For this review, take the finished solid that the model builds, in its own axes (mm). A direction names the side the tool comes from. Give positions to 0.01 mm unless a question says otherwise; leave off trailing zeros. Loops run counter-clockwise (first coordinate to the right, second up) from the corner with the lowest first, then second, coordinate; pieces in that order, holes last. Notation, with made-up numbers: (-27, -35.75) -> (2, -35.75) arc R21 ccw to (2, -2.75) -> close; hole circle Ø4 at (36.25, 52). An arc over 180 degrees is marked (long way). Answer as CSV lines item,"result". Start each with the question number.
Item 1: Machinability: for faces 1 (the face through (0, -1.5, 12)), 2 (the face through (12.93, 3.9, 11.93)), 3 (the face through (-0.147, 2.197, 2.317)), which of the approach directions +Z, -Z, +X, -X, +Y, -Y give a long, thin tool a straight path to every point of the face, cutting with its end or side? Answer none if there is none.
Item 2: For L1, parallel to Y at x = 3, z = 18; L2, parallel to Z at x = -15.5, y = -8.75; L3, parallel to Z at x = 1, y = 2, list the stretches that pass through material, from the lowest coordinate up. Write a range as from..to.
Item 3: Add section B-B on z = 15. State the section outline as (x, y) points.
Item 4: Clearance check with flat-ended pins moving along their axes: P1, Ø4, axis at x = 10, z = 15.5, coming from the +Y side; P2, Ø5, axis at y = 3, z = 6.5, coming from the +X side; P3, Ø4, axis at y = -1, z = 11.5, coming from the -X side. State where each tip first meets the part, or that it passes through.
Item 5: Add section D-D on y = 5.25. State the section outline as (x, z) points.
Item 6: The part is to be moulded in two halves that separate along Y. For faces 4 (the face through (0, 5, 0.2)), 5 (the face through (-12.93, -3.9, 11.93)), 6 (the face through (-0.147, -2.217, 22.731)), say which applies: +Y half, -Y half, draft (parallel to the pull), parting line (faces both ways), or undercut.
Item 7: Add section C-C on x = -11. State the section outline as (y, z) points, plus the area to 3 significant figures.
```python
from build123d import *

# Parameters (mm, degrees)
F0_W     = 21
F0_H     = 3
F1_DEPTH = 25
F2_SIZE  = 2
F3_SIZE  = 2
F4_R     = 0.99999
F0_W_2   = 36.543905735
F0_H_2   = 20.3890502453
F5_DEPTH = 0.2


# Not quite as in the source:
# - a fillet or chamfer is up to 0.001 mm smaller than in the source, because OpenCascade refuses the exact size


with BuildPart() as f1:
    # F0 (on Top) → F1 (new body)
    with BuildSketch(Plane.XY):
        with BuildLine():
            Line((-11.5, -4.5), (11.5, -4.5))
            ThreePointArc((11.5, -4.5), (12.9142135624, -3.9142135624), (13.5, -2.5))
            Line((13.5, -2.5), (13.5, 2.5))
            ThreePointArc((13.5, 2.5), (12.9142135624, 3.9142135624), (11.5, 4.5))
            Line((11.5, 4.5), (-11.5, 4.5))
            ThreePointArc((-11.5, 4.5), (-12.9142135624, 3.9142135624), (-13.5, 2.5))
            Line((-13.5, 2.5), (-13.5, -2.5))
            ThreePointArc((-13.5, -2.5), (-12.9142135624, -3.9142135624), (-11.5, -4.5))
        make_face()
        Rectangle(F0_W, F0_H, mode=Mode.SUBTRACT)
    extrude(amount=F1_DEPTH)

    # F2
    f2_edges = [f1.edges().sort_by_distance(p)[0] for p in [
        (0, -1.5, 25),
        (0, 1.5, 25),
        (0, 1.5, 0),
        (0, -1.5, 0),
    ]]
    chamfer(f2_edges, length=F2_SIZE)

    # F3
    f3_edges = [f1.edges().sort_by_distance(p)[0] for p in [
        (0, 1.5, 23),
        (0, -1.5, 23),
        (0, -1.5, 2),
        (0, 1.5, 2),
    ]]
    chamfer(f3_edges, length=F3_SIZE)

    # F4 (radius 1 in the source; OpenCascade refuses exactly that, so slightly less here)
    f4_edges = [f1.edges().sort_by_distance(p)[0] for p in [
        (0, 4.5, 25),
    ]]
    fillet(f4_edges, radius=F4_R)

    # F0 (on Top) → F5 (join)
    with BuildSketch(Plane.XY):
        Rectangle(F0_W_2, F0_H_2)
        with BuildLine():
            ThreePointArc((13.5, -2.5), (12.9142135624, -3.9142135624), (11.5, -4.5))
            Line((11.5, -4.5), (-11.5, -4.5))
            ThreePointArc((-11.5, -4.5), (-12.9142135624, -3.9142135624), (-13.5, -2.5))
            Line((-13.5, -2.5), (-13.5, 2.5))
            ThreePointArc((-13.5, 2.5), (-12.9142135624, 3.9142135624), (-11.5, 4.5))
            Line((-11.5, 4.5), (11.5, 4.5))
            ThreePointArc((11.5, 4.5), (12.9142135624, 3.9142135624), (13.5, 2.5))
            Line((13.5, 2.5), (13.5, -2.5))
        make_face(mode=Mode.SUBTRACT)
    extrude(amount=F5_DEPTH)


solid = f1.part
```
Computed values:
1,face 1,"+Z, -Z"
1,face 2,"+Z, +X, +Y"
1,face 3,"-Z"
2,L1,"-4.5..-1.5, 1.5..4.5"
2,L2,"0..0.2"
2,L3,"2.79..22.21"
3,outline,"(-13.5, -2.5) arc R2 ccw to (-11.5, -4.5) -> (11.5, -4.5) arc R2 ccw to (13.5, -2.5) -> (13.5, 2.5) arc R2 ccw to (11.5, 4.5) -> (-11.5, 4.5) arc R2 ccw to (-13.5, 2.5) -> close; hole (-10.5, -1.5) -> (10.5, -1.5) -> (10.5, 1.5) -> (-10.5, 1.5) -> close"
4,P1,"y = 4.5"
4,P2,"x = 13.5"
4,P3,"x = -13.5"
5,outline,"(-18.27, 0) -> (18.27, 0) -> (18.27, 0.2) -> (-18.27, 0.2) -> close"
6,face 4,"draft"
6,face 5,"-Y half"
6,face 6,"undercut"
7,outline,"(-10.19, 0) -> (10.19, 0) -> (10.19, 0.2) -> (4.5, 0.2) -> (4.5, 24) arc R1 ccw to (3.5, 25) -> (-3.5, 25) arc R1 ccw to (-4.5, 24) -> (-4.5, 0.2) -> (-10.19, 0.2) -> close"
7,area,"227 mm²"
